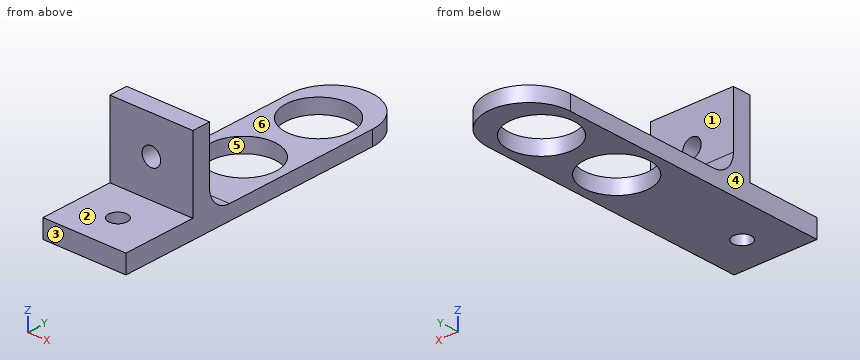
from build123d import *

# Parameters (mm, degrees)
SKETCH1_W           = 28.575
SKETCH1_H           = 76.2
SKETCH1_R           = 11.2776
BOSS_EXTRUDE1_DEPTH = 5.08
SKETCH1_3_W         = 28.575
SKETCH1_3_H         = 25.4
SKETCH1_3_R         = 3.1877
BOSS_EXTRUDE2_DEPTH = 6.35
SKETCH1_4_W         = 28.575
SKETCH1_4_H         = 6.35
BOSS_EXTRUDE3_DEPTH = 31.75
FILLET1_R           = 7.62
FILLET3_RADIUS      = 14.2875
FILLET3_LENGTH      = 5.08
SKETCH2_R           = 3.1877
CUT_EXTRUDE1_DEPTH  = 90.591839228


with BuildPart() as part:
    # Sketch1 → Boss-Extrude1 (new body)
    with BuildSketch(Plane.XY):
        with Locations((0, 15.875)):
            Rectangle(SKETCH1_W, SKETCH1_H)
        with Locations((0, 6.35)):
            Circle(SKETCH1_R, mode=Mode.SUBTRACT)
        with Locations((0, 34.925)):
            Circle(SKETCH1_R, mode=Mode.SUBTRACT)
    extrude(amount=BOSS_EXTRUDE1_DEPTH)



with BuildPart() as body_2:
    # Sketch1<3> → Boss-Extrude2 (new body)
    with BuildSketch(Plane.XY):
        with Locations((0, -41.275)):
            Rectangle(SKETCH1_3_W, SKETCH1_3_H)
        with Locations((0, -41.275)):
            Circle(SKETCH1_3_R, mode=Mode.SUBTRACT)
    extrude(amount=BOSS_EXTRUDE2_DEPTH)


with BuildPart() as part_1:
    add(part.part)

    add(body_2.part)  # Boss-Extrude3 merges body 2
    # Sketch1<4> → Boss-Extrude3 (add)
    with BuildSketch(Plane.XY):
        with Locations((0, -25.4)):
            Rectangle(SKETCH1_4_W, SKETCH1_4_H)
    extrude(amount=BOSS_EXTRUDE3_DEPTH)

    # Fillet1
    fillet1_edges = [part_1.edges().sort_by_distance(p)[0] for p in [
        (0, -22.225, 5.08),
    ]]
    fillet(fillet1_edges, radius=FILLET1_R)

    # Fillet3: full round fillet: the end face becomes a half cylinder, R = half its width
    fillet3_face = Plane((0, 53.975, 2.54), x_dir=(0, 0, 1), z_dir=(0, 1, 0))  # on the end face: x along it, z out of the body
    fillet3_slab = fillet3_face.offset(-FILLET3_RADIUS / 2) * Box(FILLET3_LENGTH, 2 * FILLET3_RADIUS, FILLET3_RADIUS, mode=Mode.PRIVATE)  # the body's end, R deep
    fillet3_round = Plane((0, 39.6875, 2.54), x_dir=(0, 1, 0), z_dir=(0, 0, 1)) * Cylinder(FILLET3_RADIUS, FILLET3_LENGTH, mode=Mode.PRIVATE)  # its axis R under the face
    add(fillet3_slab - fillet3_round, mode=Mode.SUBTRACT)

    # Sketch2 → Cut-Extrude1 (cut, through all)
    with BuildSketch(Plane.XZ.offset(28.575)):
        with Locations(Location((0, 19.05, 0), (0, 0, 270))):
            Circle(SKETCH2_R)
    extrude(amount=-CUT_EXTRUDE1_DEPTH, mode=Mode.SUBTRACT)


solid = part_1.part
Could you check a few things on this model? Use its own coordinates, in mm. Face numbers are marked on the shaded views. A direction names the side the tool comes from. Give positions to 0.01 mm unless a question says otherwise; leave off trailing zeros. Write each loop counter-clockwise with the first axis right and the second up, starting at its lowest first coordinate (ties: lowest second). Pieces come first, ordered by that corner, then holes. Notation, with made-up numbers: (-22, 4) -> (-5, 4) arc R33 cw to (-5, 33) -> close; hole circle Ø5 at (16, 21.5). An arc over 180 degrees is marked (long way). Write each question's results on one line, items separated by ' | '. Start each with the question number.
Q1. I'm going to push flat-ended pins straight in: pin 1 Ø4 at (x, z) = (-6.5, 4) entering from +Y; pin 2 Ø1.5 at (x, z) = (-4.5, 27) entering from +Y (3 decimals). Where does each tip first touch, or does it pass through?
Q2. I need wall thicknesses on probe 1 along Y at (x, z) = (0, 2.2) (3 decimals); probe 2 along X at (y, z) = (-26.25, 19.05); probe 3 along Y at (x, z) = (8, 3) (3 decimals). Which ranges of each line are inside material? Lowest first, please.
Q3. Which directions (+Z, -Z, +X, -X, +Y, -Y) give clear straight access to the entire face, cutting with the end or side of a thin tool? Please do the marked faces 1, 2 and 3.
Q4. Suppose I cut it at A-A, the plane z = 19.05. List the corners of the cut face in (x, y) for me (1 decimal).
Q5. We'd pull the mould along X, two halves only. Please class the marked faces 4, 5 and 6: +X half, -X half, draft (parallel to the pull), parting line (faces both ways), or undercut.
Q6. Suppose I cut it at C-C, the plane y = 6.35. List the corners of the cut face in (x, z) for me.
Q7. Suppose I cut it at B-B, the plane x = 0. List the corners of the cut face in (y, z) for me (3 decimals).
Q8. Suppose I cut it at D-D, the plane z = 4. State how many separate pieces and enclosed holes the cut face has, and give its area (3 significant figures).
Outcome:
1) pin 1: y = 53.25 | pin 2: y = -22.225
2) probe 1: -53.975 to -44.463, -38.087 to -4.928, 17.628 to 23.647, 46.203 to 53.975 | probe 2: -14.29 to -3.19, 3.19 to 14.29 | probe 3: -53.975 to -1.599, 14.299 to 26.976, 42.874 to 51.525
3) face 1: +Z, +X, -X, +Y | face 2: +Z, +X, -X, -Y | face 3: +Z, -Z, +X, -X, -Y
4) outline: (-14.3, -28.6) -> (-3.2, -28.6) -> (-3.2, -22.2) -> (-14.3, -22.2) -> close; (3.2, -28.6) -> (14.3, -28.6) -> (14.3, -22.2) -> (3.2, -22.2) -> close
5) face 4: -X half | face 5: undercut | face 6: draft
6) outline: (-14.29, 0) -> (-11.28, 0) -> (-11.28, 5.08) -> (-14.29, 5.08) -> close; (11.28, 0) -> (14.29, 0) -> (14.29, 5.08) -> (11.28, 5.08) -> close
7) outline: (-53.975, 0) -> (-44.463, 0) -> (-44.463, 6.35) -> (-53.975, 6.35) -> close; (-38.087, 0) -> (-4.928, 0) -> (-4.928, 5.08) -> (-14.605, 5.08) arc R7.62 cw to (-22.225, 12.7) -> (-22.225, 15.862) -> (-28.575, 15.862) -> (-28.575, 6.35) -> (-38.087, 6.35) -> close; (-28.575, 22.238) -> (-22.225, 22.238) -> (-22.225, 31.75) -> (-28.575, 31.75) -> close; (17.628, 0) -> (23.647, 0) -> (23.647, 5.08) -> (17.628, 5.08) -> close; (46.203, 0) -> (53.975, 0) -> (53.975, 5.08) -> (46.203, 5.08) -> close
8) separate pieces: 1 | enclosed holes: 3 | area: 2,170 mm2
